```python
from build123d import *
from build123d.topology import SkipClean

# Parameters (mm, degrees)
ESBO_O1_R                  = 1
RESSALTO_EXTRUS_O1_DEPTH   = 12.5
CORTE_EXTRUS_O1_DEPTH      = 15
CORTE_EXTRUS_O2_DEPTH      = 49.656962503
CORTE_EXTRUS_O2_DEPTH_BACK = 49.656962503
ESBO_O5_R                  = 1.7
RESSALTO_EXTRUS_O2_DEPTH   = 3
CORTE_EXTRUS_O3_DEPTH      = 10
CORTE_EXTRUS_O4_DEPTH      = 57.402570863
RESSALTO_EXTRUS_O3_START   = -4
RESSALTO_EXTRUS_O3_DEPTH   = 4
ESBO_O9_R                  = 5.3
CORTE_EXTRUS_O5_DEPTH      = 1.5
RESSALTO_EXTRUS_O4_DEPTH   = 0.5
CORTE_EXTRUS_O6_DEPTH      = 1.5


with BuildPart() as part:
    # Esbo_o1 → Ressalto-extrus_o1 (new, symmetric)
    with BuildSketch(Plane.XY):
        Polygon((0, -22), (-33, -22), (-33, -19), (-3, -19), (-3, 19), (-33, 19), (-33, 22), (0, 22), (13, 16.5), (13, 11.5), (0, 11.5), (0, -11.5), (13, -11.5), (13, -16.5), align=None)
        with Locations((6.5, 13.85)):
            Circle(ESBO_O1_R, mode=Mode.SUBTRACT)
        with Locations(Location((6.5, -13.85, 0), (0, 0, 180))):
            Circle(ESBO_O1_R, mode=Mode.SUBTRACT)
    extrude(amount=RESSALTO_EXTRUS_O1_DEPTH, both=True)

    # Esbo_o2 → Corte-extrus_o1 (cut)
    with BuildSketch(Plane(origin=(0, 22, 0), x_dir=(1, 0, 0), z_dir=(0, 1, 0))):
        with BuildLine():
            Line((-22.45722521, 7.240115294), (-3, 12.5))
            Line((-3, 12.5), (-33, 12.5))
            Line((-33, 12.5), (-33, -12.5))
            Line((-33, -12.5), (-3, -12.5))
            Line((-3, -12.5), (-22.45722521, -7.240115294))
            ThreePointArc((-22.45722521, -7.240115294), (-25.398129905, -5.679641136), (-27.373863542, -3))
            Line((-27.373863542, -3), (-22.75, -3))
            ThreePointArc((-22.75, -3), (-16.75, 0), (-22.75, 3))
            Line((-22.75, 3), (-27.373863542, 3))
            ThreePointArc((-27.373863542, 3), (-25.398129905, 5.679641136), (-22.45722521, 7.240115294))
        make_face()
        with BuildLine():
            Line((-5.5, 1), (-9.5, 1))
            ThreePointArc((-9.5, 1), (-10.5, 0), (-9.5, -1))
            Line((-9.5, -1), (-5.5, -1))
            ThreePointArc((-5.5, -1), (-4.5, 0), (-5.5, 1))
        make_face()
    extrude(amount=-CORTE_EXTRUS_O1_DEPTH, mode=Mode.SUBTRACT)

    # Esbo_o4 → Corte-extrus_o2 (cut, two sides: drawn at the far end of the back side and taken through both)
    with BuildSketch(Plane(origin=(0, -11.5, 0), x_dir=(1, 0, 0), z_dir=(0, 1, 0)).offset(-CORTE_EXTRUS_O2_DEPTH_BACK)):
        Polygon((13, -7.5), (0, 0.005553499), (0, 12.5), (13, 12.5), align=None)
    extrude(amount=CORTE_EXTRUS_O2_DEPTH + CORTE_EXTRUS_O2_DEPTH_BACK, mode=Mode.SUBTRACT)

    # Esbo_o5 → Ressalto-extrus_o2 (add)
    with BuildSketch(Plane(origin=(0, 0, -12.5), x_dir=(-1, 0, 0), z_dir=(0, 0, -1))):
        with BuildLine():
            Line((-8.182323793, 11.928517871), (0, 14.120964923))
            Line((0, 14.120964923), (0, -2.820964923))
            Line((0, -2.820964923), (-8.182323793, -0.628517871))
            ThreePointArc((-8.182323793, -0.628517871), (-13, 5.65), (-8.182323793, 11.928517871))
        make_face()
        with Locations((-6.5, 5.65)):
            Circle(ESBO_O5_R, mode=Mode.SUBTRACT)
    extrude(amount=-RESSALTO_EXTRUS_O2_DEPTH)

    # Esbo_o7 → Corte-extrus_o3 (cut)
    with BuildSketch(Plane(origin=(0, -19, 0), x_dir=(1, 0, 0), z_dir=(0, 1, 0))):
        with BuildLine():
            Line((-21.208872344, 1.6), (-33, 1.6))
            Line((-33, 1.6), (-33, -1.6))
            Line((-33, -1.6), (-21.208872344, -1.6))
            ThreePointArc((-21.208872344, -1.6), (-18.75, 0), (-21.208872344, 1.6))
        make_face()
    extrude(amount=-CORTE_EXTRUS_O3_DEPTH, mode=Mode.SUBTRACT)

    # Esbo_o2_2 → Corte-extrus_o4 (cut, through all)
    with BuildSketch(Plane(origin=(0, 22, 0), x_dir=(1, 0, 0), z_dir=(0, 1, 0))):
        with BuildLine():
            Line((-3, 12.5), (-22.45722521, 7.240115294))
            ThreePointArc((-22.45722521, 7.240115294), (-27.261066665, 3.246225123), (-27.373863542, -3))
            ThreePointArc((-27.373863542, -3), (-25.398129905, -5.679641136), (-22.45722521, -7.240115294))
            Line((-22.45722521, -7.240115294), (-3, -12.5))
            Line((-3, -12.5), (-33, -12.5))
            Line((-33, -12.5), (-33, 12.5))
            Line((-33, 12.5), (-3, 12.5))
        make_face()
    extrude(amount=-CORTE_EXTRUS_O4_DEPTH, mode=Mode.SUBTRACT)

    # Esbo_o8 → Ressalto-extrus_o3 (add)
    with BuildSketch(Plane(origin=(0, 0, 0), x_dir=(0, 0, -1), z_dir=(1, 0, 0)).offset(RESSALTO_EXTRUS_O3_START)):
        Polygon((10, -21.5), (3, -28.5), (-7, -28.5), (-7, -25.5), (-5, -24), (-5, -25.5), (1.757359313, -25.5), (5.757359313, -21.5), align=None)
    extrude(amount=-RESSALTO_EXTRUS_O3_DEPTH)

    # Esbo_o9 → Corte-extrus_o5 (cut)
    with BuildSketch(Plane(origin=(0, -22, 0), x_dir=(-1, 0, 0), z_dir=(0, -1, 0))):
        with Locations((20.5, 0)):
            Circle(ESBO_O9_R)
    extrude(amount=-CORTE_EXTRUS_O5_DEPTH, mode=Mode.SUBTRACT)

    # Esbo_o10 → Ressalto-extrus_o4 (add)
    with SkipClean():  # the faces are left unmerged after this step: merging them gives an invalid solid
        with BuildSketch(Plane.XZ.offset(22)):
            with BuildLine():
                Line((-27.827346041, 1.6), (-25.552722039, 1.6))
                ThreePointArc((-25.552722039, 1.6), (-15.2, 0), (-25.552722039, -1.6))
                Line((-25.552722039, -1.6), (-27.827346041, -1.6))
                ThreePointArc((-27.827346041, -1.6), (-13, 0), (-27.827346041, 1.6))
            make_face()
        extrude(amount=RESSALTO_EXTRUS_O4_DEPTH)

    # Esbo_o11 → Corte-extrus_o6 (cut)
    with SkipClean():  # the faces are left unmerged after this step: merging them gives an invalid solid
        with BuildSketch(Plane(origin=(0, 22, 0), x_dir=(1, 0, 0), z_dir=(0, 1, 0))):
            with BuildLine():
                Line((-20.088235294, 3.978749782), (-3.268382353, 2.238046752))
                ThreePointArc((-3.268382353, 2.238046752), (-1.25, 0), (-3.268382353, -2.238046752))
                Line((-3.268382353, -2.238046752), (-20.088235294, -3.978749782))
                ThreePointArc((-20.088235294, -3.978749782), (-24.5, 0), (-20.088235294, 3.978749782))
            make_face()
        extrude(amount=-CORTE_EXTRUS_O6_DEPTH, mode=Mode.SUBTRACT)


solid = part.part
```
Geometry check sheet. Reference: the model listing, model coordinates, mm. A direction names the side the tool comes from. Coordinates: 2 decimals unless noted, no trailing zeros. Loops run counter-clockwise (first coordinate to the right, second up) from the corner with the lowest first, then second, coordinate; pieces in that order, holes last.
Item 1: Sectioned sample at D-D, the plane y = -13.85. Record the boundary of the cut face in (x, z), then the cut area to 3 significant figures.
Item 2: Sectioned sample at C-C, the plane x = 6.5. Record the boundary of the cut face in (y, z).
Item 3: Thickness scan on line 1 (Y direction, x = -12, z = -5.75); line 2 (Z direction, x = 6, y = 0.5); line 3 (Y direction, x = -17, z = -6.5). Record the ranges inside material, lowest first.
Item 4: Access from +Z, -Z, +X, -X, +Y, -Y to the whole of each face (thin tool, end or side, straight path). Record for faces 1 (the face through (-25, 21, -3)), 2 (the face through (-6, -25, 5)), 3 (the face through (-13, -19, 0)).
Item 5: Sectioned sample at B-B, the plane x = -18. Record the boundary of the cut face in (y, z).
Item 6: Go/stop test with flat-tipped pins: pin 1 Ø14 at (x, z) = (5.5, 4.5) entering from -Y; pin 2 Ø3 at (x, y) = (6.5, 5.65) entering from -Z; pin 3 Ø9.5 at (x, z) = (-20.5, 0) entering from -Y; pin 4 Ø2 at (y, z) = (-2, 5) entering from +X. Record where each tip stops, or that it passes through.
Item 7: Release check for a two-part mould opening along Y. For faces 4 (the face through (-25, -20, -1.6)), 5 (the face through (13, 5.5, -11)), 6 (the face through (6.721, 7.336, -11.021)) record: released by +Y, released by -Y, zero draft, split by the parting line, or undercut.
Item 8: Sectioned sample at A-A, the plane y = 5.65. Record the boundary of the cut face in (x, z).
Check result:
1. outline: (-3, -12.5) - (0, -12.5) - (0, -0.01) - (5.5, 3.17) - (5.5, 12.5) - (-3, 12.5) - close; (7.5, 4.32) - (13, 7.5) - (13, 12.5) - (7.5, 12.5) - close
1. area: 171 mm2
2. outline: (-19.25, 3.75) - (-14.85, 3.75) - (-14.85, 12.5) - (-19.25, 12.5) - close; (-12.85, 3.75) - (-11.5, 3.75) - (-11.5, 12.5) - (-12.85, 12.5) - close; (-1.08, -12.5) - (3.95, -12.5) - (3.95, -9.5) - (-1.08, -9.5) - close; (7.35, -12.5) - (12.38, -12.5) - (12.38, -9.5) - (7.35, -9.5) - close; (11.5, 3.75) - (12.85, 3.75) - (12.85, 12.5) - (11.5, 12.5) - close; (14.85, 3.75) - (19.25, 3.75) - (19.25, 12.5) - (14.85, 12.5) - close
3. line 1: y = -22 to -19, 19 to 22
3. line 2: z = -12.5 to -9.5
3. line 3: y = -22.5 to -19, 19 to 22
4. face 1: -X, +Y
4. face 2: +X, -X
4. face 3: +Z, -Z, -X
5. outline: (-22.5, -7.07) - (-22, -7.07) - (-22, -8.45) - (-19, -8.45) - (-19, 8.45) - (-22, 8.45) - (-22, 7.07) - (-22.5, 7.07) - (-22.5, 4.67) - (-20.5, 4.67) - (-20.5, -4.67) - (-22.5, -4.67) - close; (19, -8.45) - (22, -8.45) - (22, -3.76) - (20.5, -3.76) - (20.5, -2.8) - (19, -2.8) - close; (19, 2.8) - (20.5, 2.8) - (20.5, 3.76) - (22, 3.76) - (22, 8.45) - (19, 8.45) - close
6. pin 1: stops at y = -22
6. pin 2: passes through
6. pin 3: stops at y = -20.5
6. pin 4: stops at x = 0
7. face 4: zero draft
7. face 5: split by the parting line
7. face 6: undercut
8. outline: (-3, -12.5) - (4.8, -12.5) - (4.8, -9.5) - (0, -9.5) - (0, 12.5) - (-3, 12.5) - close; (8.2, -12.5) - (13, -12.5) - (13, -9.5) - (8.2, -9.5) - close
